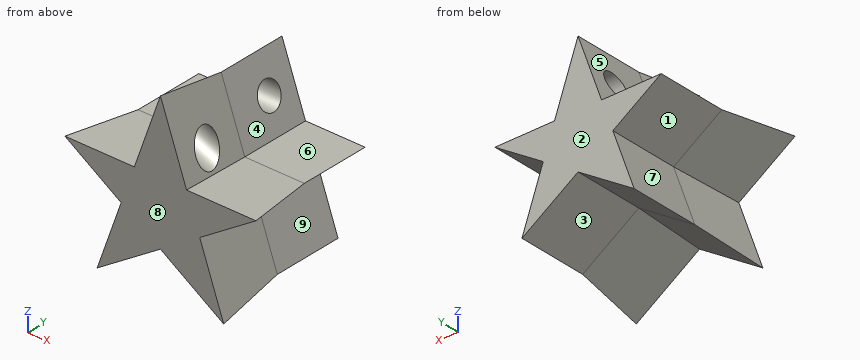
```python
from build123d import *

# Parameters (mm, degrees)
F2_DEPTH      = 12.7
F2_TAPER      = -3
F2_DEPTH_BACK = 12.7
F3_R          = 2.54
F4_DEPTH      = 8.0921539509
F5_R          = 2.3034089063
F6_DEPTH      = 27.362293552


with BuildPart() as f2:
    # F1 (on Front) → F2 (new body, two sides)
    with BuildSketch(Plane.XZ) as f2_sk:
        Polygon((-16.4084644725, 10.7080111944), (-20.2470514737, 0), (-10.1235257369, 6.606518672), align=None)
        Polygon((-25.1235257369, 16.3953790609), (-16.4084644725, 10.7080111944), (-14.3696679147, 16.3953790609), align=None)
        Polygon((-14.3696679147, 16.3953790609), (-16.4084644725, 10.7080111944), (-10.1235257369, 6.606518672), (-3.8385870012, 10.7080111944), (-5.877383559, 16.3953790609), align=None)
        Polygon((-3.8385870012, 10.7080111944), (-10.1235257369, 6.606518672), (0, 0), align=None)
        Polygon((-10.1235257369, 28.2402943798), (-14.3696679147, 16.3953790609), (-5.877383559, 16.3953790609), align=None)
        Polygon((-5.877383559, 16.3953790609), (-3.8385870012, 10.7080111944), (4.8764742631, 16.3953790609), align=None)
    extrude(amount=F2_DEPTH, taper=F2_TAPER)
    extrude(f2_sk.sketch, amount=-F2_DEPTH_BACK)

    # F3 (on face) → F4 (cut, through all)
    with BuildSketch(Plane(origin=(-17.892314741, 0.9961261053, 6.4140021466), x_dir=(-0.0492660937, -0.9986295348, 0.0176608133), z_dir=(-0.9400530679, 0.0523359562, 0.3369883932))):
        with Locations((7.3562075321, 16.8761180249)):
            Circle(F3_R)
    extrude(amount=-F4_DEPTH, mode=Mode.SUBTRACT)

    # F5 (on Right) → F6 (cut, through all)
    with BuildSketch(Plane.YZ):
        with Locations((7.44647393, 22.0010466874)):
            Circle(F5_R)
    extrude(amount=-F6_DEPTH, mode=Mode.SUBTRACT)


solid = f2.part
```
Here's how the part is built. I have some questions about the finished solid (model axes, mm). Face numbers are marked on the shaded views. A direction names the side the tool comes from. Coordinates: 2 decimals unless noted, no trailing zeros. Write each loop counter-clockwise with the first axis right and the second up, starting at its lowest first coordinate (ties: lowest second). Pieces come first, ordered by that corner, then holes. Notation, with made-up numbers: M 5,58.5 L 24,58.5 A28 cw 24,95.5 Z; hole C 1,31 d7. An arc over 180 degrees is marked long. Answer as CSV lines item,"result". Start each with the question number.
Q1. For the marked faces 5, 6, 7, 8 and 9, which set-ups out of +Z, -Z, +X, -X, +Y, -Y let a thin tool reach every point of the face, with its end or its side?
Q2. Suppose I cut it at C-C, the plane x = -9. State how many separate pieces and enclosed holes the cut face has, then the cut area to 3 significant figures.
Q3. Will these pins go through, and if not, where does the flat tip stop? pin 1 Ø4 at (y, z) = (7.45, 22) entering from +X; pin 2 Ø6 at (y, z) = (-3.5, 22) entering from -X; pin 3 Ø1 at (x, y) = (-20, -3.5) entering from +Z (3 decimals).
Q4. Suppose I cut it at B-B, the plane y = 7. List the corners of the cut face in (x, z) for me.
Q5. Suppose I cut it at A-A, the plane y = 0.75. List the corners of the cut face in (x, z) for me, then the cut area to 3 significant figures.
Q6. I need wall thicknesses on probe 1 along X at (y, z) = (8, 2); probe 2 along X at (y, z) = (-10.75, 25); probe 3 along Y at (x, z) = (-8.5, 18.5). Which ranges of each line are inside material? Lowest first, please. Write a range as [from, to].
Q7. If we mould it in two halves opening along Z, with no side actions, what happens to the marked faces 1, 2, 3 and 4? For each: pulls with the +Z half, pulls with the -Z half, needs draft (parallel to the pull), parting line crosses it, or undercut.
Entries:
1,face 5,"+Z, -X, +Y"
1,face 6,"+Z, +X, +Y"
1,face 7,"-X, +Y"
1,face 8,"+Z, -Z, +X, -X, -Y"
1,face 9,"+X, +Y"
2,separate pieces,"1"
2,enclosed holes,"2"
2,area,"468 mm²"
3,pin 1,"passes through"
3,pin 2,"stops at x = -13.64"
3,pin 3,"stops at z = 16.605"
4,outline,"M -25.12,16.4 L -16.41,10.71 L -20.25,0 L -10.12,6.61 L 0,0 L -3.84,10.71 L 4.88,16.4 L -5.88,16.4 L -7.08,19.74 L -13.17,19.74 L -14.37,16.4 Z; M -11.55,24.26 L -8.7,24.26 L -10.12,28.24 Z"
5,outline,"M -25.12,16.4 L -16.41,10.71 L -20.25,0 L -10.12,6.61 L 0,0 L -3.84,10.71 L 4.88,16.4 L -5.88,16.4 L -10.12,28.24 L -14.37,16.4 Z"
5,area,"280 mm²"
6,probe 1,"x = [-19.53, -17.18], [-3.06, -0.72]"
6,probe 2,"x = [-11.88, -8.36]"
6,probe 3,"y = [-12.7, -7.63], [-5.61, 12.7]"
7,face 1,"undercut"
7,face 2,"needs draft"
7,face 3,"pulls with the -Z half"
7,face 4,"pulls with the +Z half"
